Geometry: final body of the model. Coordinates: model frame, mm. Round coordinates to 2 decimals unless told otherwise and drop trailing zeros. Loops run counter-clockwise (first coordinate to the right, second up) from the corner with the lowest first, then second, coordinate; pieces in that order, holes last. Notation, with made-up numbers: M -3.75,-23.75 L 51.25,-23.75 A26 ccw 51.25,-6.75 Z; hole C 27,21 d9. An arc over 180 degrees is marked long. Answer as a JSON object with one key per item and string values.
from build123d import *

# Parameters (mm, degrees)
SKETCH1_W         = 210
SKETCH1_H         = 210
MAINEXTRUDE_DEPTH = 4
SKETCH1_6_R       = 1.5
SCREWHOLES_DEPTH  = 4
ROUNDEDCORNERS_R  = 10
SKETCH3_R         = 7
TRENCH_DEPTH      = 4


with BuildPart() as part:
    # Sketch1 → MainExtrude (new body)
    with BuildSketch(Plane(origin=(0, 0, 0), x_dir=(1, 0, 0), z_dir=(0, 1, 0))):
        Rectangle(SKETCH1_W, SKETCH1_H)
    extrude(amount=MAINEXTRUDE_DEPTH)

    # Sketch1<6> → ScrewHoles (cut)
    with BuildSketch(Plane(origin=(0, 0, 0), x_dir=(1, 0, 0), z_dir=(0, 1, 0))):
        with Locations((-99.833273811, 99.833273811)):
            Circle(SKETCH1_6_R)
        with Locations((-99.833273811, -99.833273811)):
            Circle(SKETCH1_6_R)
        with Locations((99.833273811, -99.833273811)):
            Circle(SKETCH1_6_R)
        with Locations((99.833273811, 99.833273811)):
            Circle(SKETCH1_6_R)
    extrude(amount=SCREWHOLES_DEPTH, mode=Mode.SUBTRACT)

    # RoundedCorners
    roundedcorners_edges = [part.edges().sort_by_distance(p)[0] for p in [
        (-105, 2, -105),
        (-105, 2, 105),
        (105, 2, 105),
        (105, 2, -105),
    ]]
    fillet(roundedcorners_edges, radius=ROUNDEDCORNERS_R)

    # Sketch3 → Trench (cut)
    with BuildSketch(Plane(origin=(0, 0, 0), x_dir=(1, 0, 0), z_dir=(0, 1, 0))):
        with Locations((-52.205723714, -65.868416485)):
            Circle(SKETCH3_R)
        Polygon((-38, 90), (-38, 39), (-90, 39), (-90, 29), (2, 29), (2, -39), (-80, -39), (-80, -9), (-22, -9), (-22, 1), (-90, 1), (-90, -49), (-41, -49), (-41, -93), (95, -93), (95, -39), (49, -39), (49, 1), (90, 1), (90, 96), (80, 96), (80, 11), (39, 11), (39, -39), (27, -39), (27, -49), (85, -49), (85, -83), (-31, -83), (-31, -49), (12, -49), (12, 39), (-28, 39), (-28, 90), align=None)
    extrude(amount=TRENCH_DEPTH, mode=Mode.SUBTRACT)


solid = part.part
1) Section query D-D (y = 1.85). Count the separate pieces of the cut face and the enclosed holes in it, and give its area (3 significant figures).
Results:
{"separate pieces": "1", "enclosed holes": "6", "area": "35,100 mm2"}
2) Pull-direction query (Z, two-part tool) for faces 1 (the flat face through (-1, 4, -25)), 2 (the cylindrical face through (-53.12, 1.97, 58.93)), 3 (the cylindrical face through (101.99, 2.03, -102.15)); classes: +Z half, -Z half, draft (parallel to the pull), parting line (faces both ways), or undercut.
Results:
{"face 1": "draft", "face 2": "undercut", "face 3": "-Z half"}
3) Ray query, line 1 (X direction, y = 0.35, z = -21.5); line 2 (Z direction, x = 37, y = 3); line 3 (X direction, y = 1.55, z = -63). Return the intervals inside material, ascending.
Results:
{"line 1": "-105 to 2, 12 to 80, 90 to 105", "line 2": "-105 to 39, 49 to 83, 93 to 105", "line 3": "-105 to -38, -28 to 80, 90 to 105"}
4) Pin query (flat end, axial travel): P1, Ø5, axis at x = -19, z = -36, coming from the +Y side. Return the tip coordinate at first contact, or that it passes through.
Results:
{"P1": "through"}
5) Section query B-B (z = 87). Return the cut outline in (x, y), and give its area (3 significant figures).
Results:
{"outline": "M -105,0 L -41,0 L -41,4 L -105,4 Z; M 95,0 L 105,0 L 105,4 L 95,4 Z", "area": "296 mm2"}
6) Section query C-C (x = -66.5). Return the cut outline in (y, z).
Results:
{"outline": "M 0,-105 L 4,-105 L 4,-39 L 0,-39 Z; M 0,-29 L 4,-29 L 4,-1 L 0,-1 Z; M 0,9 L 4,9 L 4,39 L 0,39 Z; M 0,49 L 4,49 L 4,105 L 0,105 Z"}
7) Section query A-A (x = 36). Return the cut outline in (y, z), and give its area (3 significant figures).
Results:
{"outline": "M 0,-105 L 4,-105 L 4,39 L 0,39 Z; M 0,49 L 4,49 L 4,83 L 0,83 Z; M 0,93 L 4,93 L 4,105 L 0,105 Z", "area": "760 mm2"}
